from build123d import *

# Parameters (mm, degrees)
SKETCH_1_W             = 90
SKETCH_1_H             = 27
EXTRUDE_1_DEPTH        = 45
SKETCH_2_W             = 30
SKETCH_2_H             = 26
CUT_EXTRUDE_1_DEPTH    = 66.055745327
HOLE_WIZARD_M6_1_D     = 5
HOLE_WIZARD_M6_1_DEPTH = 11
HOLE_WIZARD_M6_1_TIP   = 1.502151548
SKETCH_6_R             = 6
EXTRUDE_2_DEPTH        = 10
EXTRUDE_3_DEPTH        = 6


with BuildPart() as part:
    # 草图1 → 凸台-拉伸1 (new body)
    with BuildSketch(Plane.XY):
        Rectangle(SKETCH_1_W, SKETCH_1_H)
    extrude(amount=EXTRUDE_1_DEPTH)

    # 草图2 → 切除-拉伸1 (cut, through all)
    with BuildSketch(Plane.XY.offset(45)):
        with Locations((0, -13.5)):
            Rectangle(SKETCH_2_W, SKETCH_2_H)
    extrude(amount=-CUT_EXTRUDE_1_DEPTH, mode=Mode.SUBTRACT)

    # M6 螺纹孔1
    with Locations(Plane(origin=(0, 13.5, 0), x_dir=(1, 0, 0), z_dir=(0, 1, 0))):
        with Locations((-14, -8.5), (14, -8.5), (14, -36.5), (-14, -36.5)):
            Hole(HOLE_WIZARD_M6_1_D / 2, depth=HOLE_WIZARD_M6_1_DEPTH)
            with Locations((0, 0, -(HOLE_WIZARD_M6_1_DEPTH + HOLE_WIZARD_M6_1_TIP / 2))):  # 118° drill point
                Cone(0, HOLE_WIZARD_M6_1_D / 2, HOLE_WIZARD_M6_1_TIP, mode=Mode.SUBTRACT)

    # 草图6 → 凸台-拉伸2 (add)
    with BuildSketch(Plane.ZY.offset(45)):
        with Locations((22.5, 4.5)):
            Circle(SKETCH_6_R)
    extrude(amount=EXTRUDE_2_DEPTH)

    # 草图8 → 凸台-拉伸3 (add, symmetric)
    with BuildSketch(Plane(origin=(0, 4.5, 0), x_dir=(1, 0, 0), z_dir=(0, 1, 0))):
        Polygon((-55, -32.420186034), (-55, -12.579813966), (-92.527767497, 32.579813966), (-100.527767497, 32.579813966), (-63, -32.420186034), align=None)
    extrude(amount=EXTRUDE_3_DEPTH, both=True)


solid = part.part
Design review of the part built by this model. Coordinates are the model's own, in mm. A direction names the side the tool comes from. Coordinates: 2 decimals unless noted, no trailing zeros. Loops run counter-clockwise (first coordinate to the right, second up) from the corner with the lowest first, then second, coordinate; pieces in that order, holes last.
Item 1: For faces 4 (the cylindrical face through (-12, 8, 10)), 5 (the flat face through (-59, 5, 32.42)), 6 (the flat face through (-55, 5, 15)), list the 3-axis set-ups (+Z, -Z, +X, -X, +Y, -Y) from which the entire face can be reached by the end or side of a thin tool; tool diameter is ignored.
Completed:
face 4: +Y
face 5: +Z, -X, +Y, -Y
face 6: -Z
Item 2: Add section B-B (y = 4.5). Write out the cut boundary in (x, z), and give its area (3 significant figures).
Completed:
outline: (-100.53, -32.58) - (-92.53, -32.58) - (-55, 12.58) - (-55, 16.5) - (-45, 16.5) - (-45, 0) - (45, 0) - (45, 45) - (-45, 45) - (-45, 28.5) - (-55, 28.5) - (-55, 32.42) - (-63, 32.42) - close; hole circle Ø5 at (-14, 8.5); hole circle Ø5 at (-14, 36.5); hole circle Ø5 at (14, 8.5); hole circle Ø5 at (14, 36.5)
area: 4,980 mm2
Item 3: Clearance check with flat-ended pins moving along their axes: pin 1 (2 mm diameter, centred on x = -69, z = 13.5, fed in from +Y); pin 2 (3 mm diameter, centred on y = 1.5, z = -14.5, fed in from +X); pin 3 (4.5 mm diameter, centred on x = 14, z = 36.5, fed in from +Y); pin 4 (6.5 mm diameter, centred on x = 14, z = 8.5, fed in from -Y). State where each tip first meets the part, or that it passes through.
Completed:
pin 1: stops at y = 10.5
pin 2: stops at x = -76.26
pin 3: stops at y = 2.35
pin 4: stops at y = -13.5
Item 4: Wall thickness on L1, parallel to Z at x = -14, y = 5.5; L2, parallel to X at y = 7, z = 36.5; L3, parallel to X at y = -1.25, z = 1: over which ranges is each line inside the solid? List them lowest first.
Completed:
L1: z = 0 to 6, 11 to 34, 39 to 45
L2: x = -45 to -16.5, -11.5 to 11.5, 16.5 to 45
L3: x = -81.14 to -64.62, -45 to -15, 15 to 45
Item 5: Add section A-A (y = -7.5). Write out the cut boundary in (x, z), and give its area (3 significant figures).
Completed:
outline: (-45, 0) - (-15, 0) - (-15, 45) - (-45, 45) - close; (15, 0) - (45, 0) - (45, 45) - (15, 45) - close
area: 2,700 mm2
Item 6: Add section D-D (x = -20.5). Write out the cut boundary in (y, z), and give its area (4 significant figures).
Completed:
outline: (-13.5, 0) - (13.5, 0) - (13.5, 45) - (-13.5, 45) - close
area: 1,215 mm2
Item 7: Add section C-C (z = 3). Write out the cut boundary in (x, y), and give its area (3 significant figures).
Completed:
outline: (-79.99, -1.5) - (-62.96, -1.5) - (-62.96, 10.5) - (-79.99, 10.5) - close; (-45, -13.5) - (-15, -13.5) - (-15, -0.5) - (15, -0.5) - (15, -13.5) - (45, -13.5) - (45, 13.5) - (-45, 13.5) - close
area: 2,240 mm2
Item 8: Draft analysis for pull direction Z (two halves, no side actions). For faces 1 (the flat face through (-73.5, 4.58, -9.68)), 2 (the flat face through (-55, 5, 30)), 3 (the conical face through (-14.434, 1.259, 36.481)), state which applies: pulls with the +Z half, pulls with the -Z half, needs draft (parallel to the pull), parting line crosses it, or undercut.
Completed:
face 1: pulls with the -Z half
face 2: needs draft
face 3: undercut
